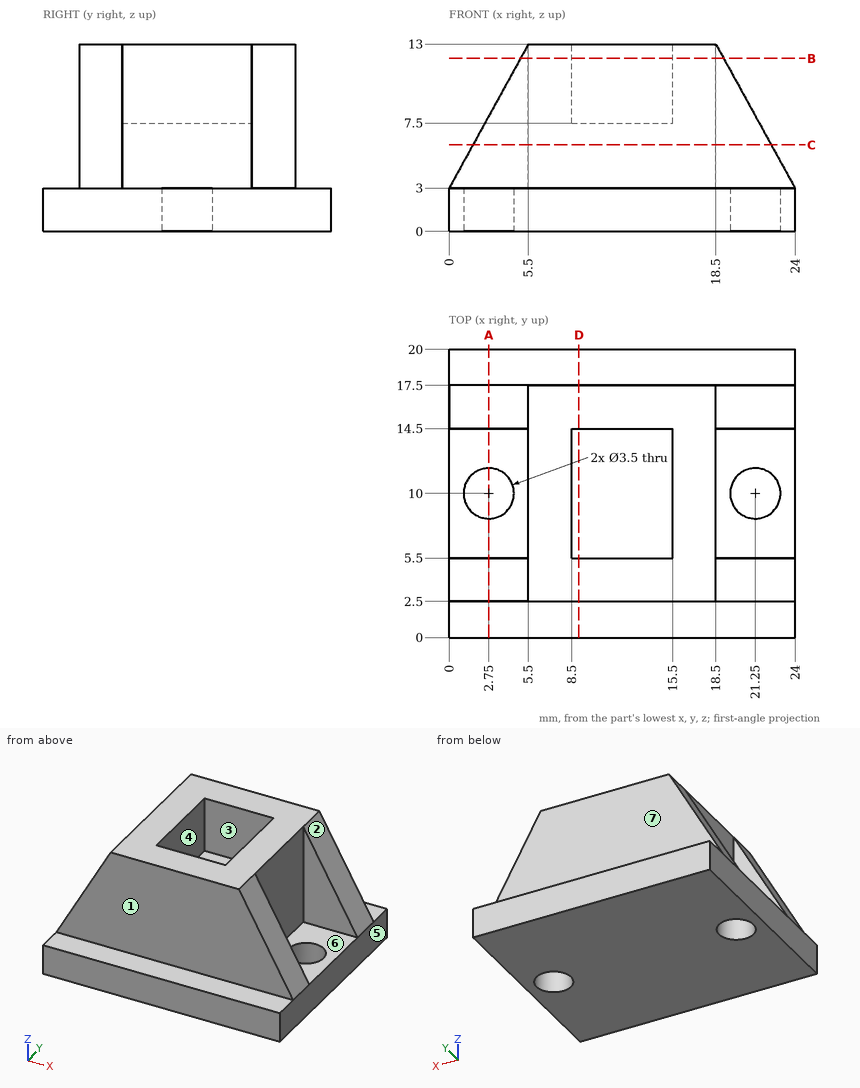
Job drawing, mm, ordinate dimensions from the low corner. One solid piece. A direction names the side the tool comes from. Give positions to 0.01 mm unless a question says otherwise; leave off trailing zeros. Loops run counter-clockwise (first coordinate to the right, second up) from the corner with the lowest first, then second, coordinate; pieces in that order, holes last. Notation, with made-up numbers: (57.25, 75) -> (88.25, 75) arc R33 ccw to (88.25, 105) -> close; hole circle Ø3 at (58.25, -28). An arc over 180 degrees is marked (long way). Write each question's results on one line, items separated by ' | '.
(1) Cut at B-B on z = 12. List the corners of the cut face in (x, y), and give its area (3 significant figures).
Geometry results:
outline: (4.95, 2.5) -> (19.05, 2.5) -> (19.05, 5.5) -> (18.5, 5.5) -> (18.5, 14.5) -> (19.05, 14.5) -> (19.05, 17.5) -> (4.95, 17.5) -> (4.95, 14.5) -> (5.5, 14.5) -> (5.5, 5.5) -> (4.95, 5.5) -> close; hole (8.5, 5.5) -> (15.5, 5.5) -> (15.5, 14.5) -> (8.5, 14.5) -> close | area: 139 mm²
(2) Probe line 1 along Y through (x, z) = (2.75, 1.75); line 2 along Y through (x, z) = (4.75, 6); line 3 along X through (y, z) = (9, 1.5). List the from-to ranges inside material, lowest first.
Geometry results:
line 1: y = 0 to 8.25, 11.75 to 20 | line 2: y = 2.5 to 5.5, 14.5 to 17.5 | line 3: x = 0 to 1.31, 4.19 to 19.81, 22.69 to 24
(3) Pull direction Y, two halves, no side cores. Call the marked faces 1, 2 and 3: released by +Y, released by -Y, zero draft, split by the parting line, or undercut.
Geometry results:
face 1: released by -Y | face 2: zero draft | face 3: undercut
(4) Cut at D-D on x = 9. List the corners of the cut face in (y, z).
Geometry results:
outline: (0, 0) -> (20, 0) -> (20, 3) -> (17.5, 3) -> (17.5, 13) -> (14.5, 13) -> (14.5, 7.5) -> (5.5, 7.5) -> (5.5, 13) -> (2.5, 13) -> (2.5, 3) -> (0, 3) -> close
(5) Cut at C-C on z = 6. List the corners of the cut face in (x, y).
Geometry results:
outline: (1.65, 2.5) -> (22.35, 2.5) -> (22.35, 5.5) -> (18.5, 5.5) -> (18.5, 14.5) -> (22.35, 14.5) -> (22.35, 17.5) -> (1.65, 17.5) -> (1.65, 14.5) -> (5.5, 14.5) -> (5.5, 5.5) -> (1.65, 5.5) -> close
(6) Flat gauge pins, fed straight in: pin 1 Ø4.5 at (x, z) = (22, 10) entering from +Y; pin 2 Ø4.5 at (y, z) = (11, 6) entering from +X; pin 3 Ø4.5 at (x, z) = (2, 6.5) entering from -Y; pin 4 Ø8 at (x, y) = (2.5, 15) entering from -Z. Where does each tip first touch, or does it go through?
Geometry results:
pin 1: stops at y = 17.5 | pin 2: stops at x = 18.5 | pin 3: stops at y = 2.5 | pin 4: stops at z = 0
(7) Tool access for the marked faces 4, 5, 6 and 7: list every direction of +Z, -Z, +X, -X, +Y, -Y with a clear straight run to the whole face (end or side of a thin tool).
Geometry results:
face 4: +Z | face 5: +Z, -Z, +X, +Y, -Y | face 6: +Z, +X | face 7: +Z, +X, -X, +Y
(8) Cut at A-A on x = 2.75. List the corners of the cut face in (y, z), and give its area (3 significant figures).
Geometry results:
outline: (0, 0) -> (8.25, 0) -> (8.25, 3) -> (5.5, 3) -> (5.5, 8) -> (2.5, 8) -> (2.5, 3) -> (0, 3) -> close; (11.75, 0) -> (20, 0) -> (20, 3) -> (17.5, 3) -> (17.5, 8) -> (14.5, 8) -> (14.5, 3) -> (11.75, 3) -> close | area: 79.5 mm²
